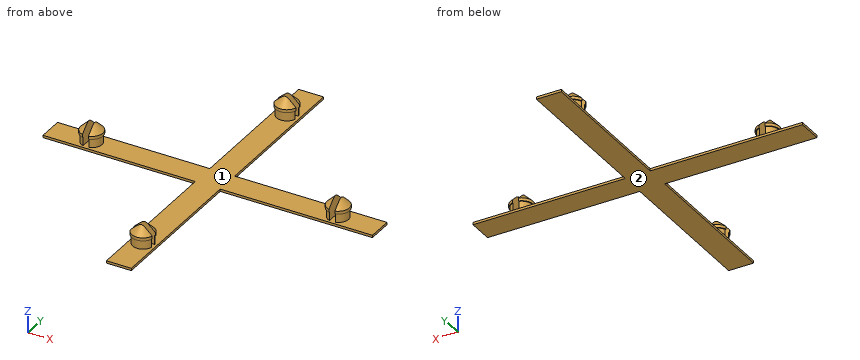
from build123d import *

# Parameters (mm, degrees)
SKICA2_W                 = 4.2
SKICA2_H                 = 55.6
SKICA2_W_2               = 55.6
SKICA2_H_2               = 4.2
P_IDAT_VYSUNUT_M2_DEPTH  = 0.4
SKICA3_R                 = 1.75
P_IDAT_VYSUNUT_M3_DEPTH  = 1.5
SKICA5_R                 = 1.9
P_IDAT_VYSUNUT_M5_DEPTH  = 2
ZKOSEN_2_SIZE            = 1.5
SKICA7_W                 = 1
SKICA7_H                 = 5
SKICA7_W_2               = 5
SKICA7_H_2               = 1
ODEBRAT_VYSUNUT_M1_DEPTH = 3.5


with BuildPart() as part:
    # Skica2 → Přidat vysunutím2 (new body)
    with BuildSketch(Plane.XY):
        Rectangle(SKICA2_W, SKICA2_H)
        Rectangle(SKICA2_W_2, SKICA2_H_2)
    extrude(amount=P_IDAT_VYSUNUT_M2_DEPTH)

    # Skica3 → Přidat vysunutím3 (add)
    with BuildSketch(Plane.XY.offset(0.4)):
        with Locations((-20.8, 0)):
            Circle(SKICA3_R)
        with Locations((0, 20.8)):
            Circle(SKICA3_R)
        with Locations((20.8, 0)):
            Circle(SKICA3_R)
        with Locations((0, -20.8)):
            Circle(SKICA3_R)
    extrude(amount=P_IDAT_VYSUNUT_M3_DEPTH)

    # Skica5 → Přidat vysunutím5 (add)
    with BuildSketch(Plane.XY.offset(1.9)):
        with Locations((-20.8, 0)):
            Circle(SKICA5_R)
        with Locations((20.8, 0)):
            Circle(SKICA5_R)
        with Locations((0, 20.8)):
            Circle(SKICA5_R)
        with Locations((0, -20.8)):
            Circle(SKICA5_R)
    extrude(amount=P_IDAT_VYSUNUT_M5_DEPTH)

    # Zkosení2
    zkosen_2_edges = [part.edges().sort_by_distance(p)[0] for p in [
        (-1.9, 20.8, 3.9),
        (-22.7, 0, 3.9),
        (18.9, 0, 3.9),
        (-1.9, -20.8, 3.9),
    ]]
    chamfer(zkosen_2_edges, length=ZKOSEN_2_SIZE)

    # Skica7 → Odebrat vysunutím1 (cut)
    with BuildSketch(Plane.XY.offset(3.9)):
        with Locations((-20.8, 0)):
            Rectangle(SKICA7_W, SKICA7_H)
        with Locations((20.8, 0)):
            Rectangle(SKICA7_W, SKICA7_H)
        with Locations((0, -20.8)):
            Rectangle(SKICA7_W_2, SKICA7_H_2)
        with Locations((0, 20.8)):
            Rectangle(SKICA7_W_2, SKICA7_H_2)
    extrude(amount=-ODEBRAT_VYSUNUT_M1_DEPTH, mode=Mode.SUBTRACT)


solid = part.part
For this review, take the finished solid that the model builds, in its own axes (mm). Face numbers are marked on the shaded views. Give positions to 0.01 mm unless a question says otherwise; leave off trailing zeros. Loops run counter-clockwise (first coordinate to the right, second up) from the corner with the lowest first, then second, coordinate; pieces in that order, holes last. Notation, with made-up numbers: (86, 84) -> (96, 84) arc R14 ccw to (96, 91) -> close; hole circle Ø2 at (20.25, 19.5). An arc over 180 degrees is marked (long way). One line per question, with ' | ' between items.
1) We need section A-A (y = 13). Write out the cut boundary in (x, z).
Resolved:
outline: (-2.1, 0) -> (2.1, 0) -> (2.1, 0.4) -> (-2.1, 0.4) -> close
2) Insertion check: pin 1 Ø1.7 at (x, z) = (1, 1.5) entering from +Y; pin 2 Ø1 at (x, z) = (21, 0.5) entering from +Y; pin 3 Ø1.7 at (y, z) = (0.5, 2.5) entering from +X. Each pin has a flat end and moves straight along its axis. Give the tip position at first contact, or say it passes through.
Resolved:
pin 1: stops at y = 22.68 | pin 2: stops at y = 2.1 | pin 3: stops at x = 22.7
3) To check wall thickness, follow probe 1 along Z at (x, y) = (-12, 0); probe 2 along Y at (x, z) = (18, 0.25). State the ranges of each line that lie inside material, in increasing order.
Resolved:
probe 1: z = 0 to 0.4 | probe 2: y = -2.1 to 2.1
4) The part is to be moulded in two halves that separate along X. For the marked faces 1 and 2, say which applies: +X half, -X half, draft (parallel to the pull), parting line (faces both ways), or undercut.
Resolved:
face 1: undercut | face 2: draft
